Input: part model. Units: mm. Frame: model coordinates. Face numbers are marked on the shaded views. A direction names the side the tool comes from. Coordinates: 2 decimals unless noted, no trailing zeros.
1) Section query A-A (y = 2.5). State how many separate pieces and enclosed holes the cut face has, then the cut area to 3 significant figures.
2) Pin query (flat end, axial travel): pin 1 Ø1.6 at (y, z) = (1, -5.5) entering from -X; pin 2 Ø1.6 at (y, z) = (1.5, -4.5) entering from +X; pin 3 Ø1 at (y, z) = (2, 4) entering from -X. Return the tip coordinate at first contact, or that it passes through.
3) Set-up query: the marked faces 3 and 4. Return all of +Z, -Z, +X, -X, +Y, -Y with unobstructed straight access to the full face (end or side cutting, diameter ignored); none if empty.
4) Line query: L1, parallel to Z at x = -0.5, y = 0.2 (3 decimals); L2, parallel to X at y = 1.3, z = 11; L3, parallel to X at y = 0.45, z = -4.25. Output: solid intervals per line, ascending.
5) Draft query along X for the marked faces 1 and 2. Return one class per face: pulls with the +X half, pulls with the -X half, needs draft (parallel to the pull), parting line crosses it, or undercut.
from build123d import *

# Parameters (mm, degrees)
SKETCH1_RX          = 12.7
SKETCH1_RY          = 6.35
BOSS_EXTRUDE1_DEPTH = 3.175
SKETCH2_W           = 3.175
SKETCH2_H           = 3.175
CUT_EXTRUDE1_DEPTH  = 4.175


with BuildPart() as part:
    # Sketch1 → Boss-Extrude1 (new body)
    with BuildSketch(Plane(origin=(0, 0, 0), x_dir=(1, 0, 0), z_dir=(0, 1, 0))):
        with Locations(Location((0, 0), (0, 0, 90))):
            Ellipse(SKETCH1_RX, SKETCH1_RY)
    extrude(amount=BOSS_EXTRUDE1_DEPTH)

    # Sketch2 → Cut-Extrude1 (cut, through all)
    with BuildSketch(Plane(origin=(0, 3.175, 0), x_dir=(1, 0, 0), z_dir=(0, 1, 0))):
        with Locations((0, 4.7675)):
            Rectangle(SKETCH2_W, SKETCH2_H)
        with Locations((0, -4.7625)):
            Rectangle(SKETCH2_W, SKETCH2_H)
    extrude(amount=-CUT_EXTRUDE1_DEPTH, mode=Mode.SUBTRACT)


solid = part.part
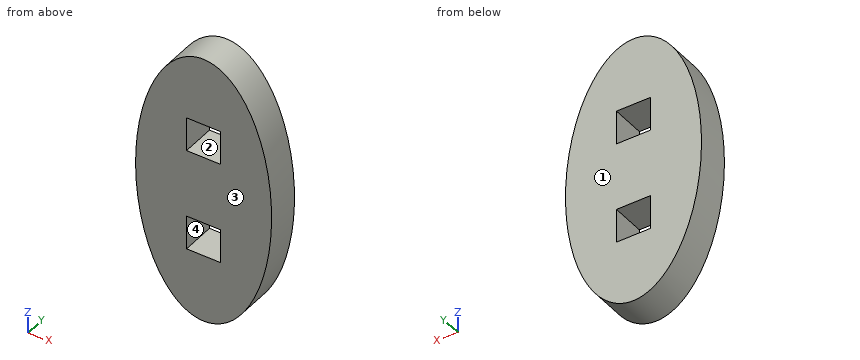
Answer:
1. separate pieces: 1
1. enclosed holes: 2
1. area: 233 mm2
2. pin 1: stops at x = -5.9
2. pin 2: stops at x = 6.07
2. pin 3: stops at x = -6.1
3. face 3: +Z, -Z, +X, -X, -Y
3. face 4: +Y, -Y
4. L1: z = -12.661 to -6.355, -3.18 to 3.175, 6.35 to 12.661
4. L2: x = -3.17 to 3.17
4. L3: x = -5.98 to -1.59, 1.59 to 5.98
5. face 1: needs draft
5. face 2: undercut
